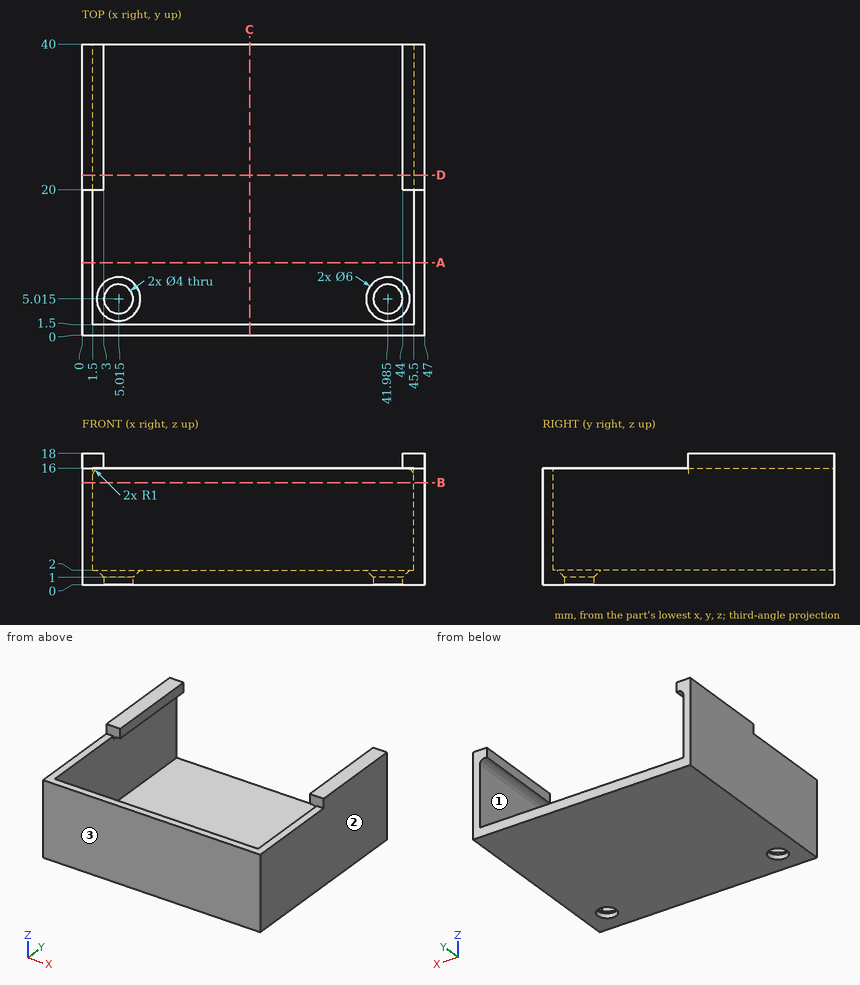
Design review of the part shown in the three views and the two pictorial views. Dimensions are in mm from the part's minimum x, y and z. Round coordinates to 2 decimals unless told otherwise and drop trailing zeros. Order: outer loops, then holes, each group sorted by start corner. A loop starts at its lowest first (then second) coordinate and runs counter-clockwise, first axis right, second up. Notation, with made-up numbers: M -14,-23.5 L 37,-23.5 A20 cw 37,13.5 Z; hole C 1.5,-10 d11. An arc over 180 degrees is marked long. Put each result on its own line as item: value.
Q1. To check wall thickness, follow line 1 (X direction, y = 8.5, z = 7.75); line 2 (Z direction, x = 4.5, y = 9); line 3 (Y direction, x = 30, z = 3.25). State the ranges of each line that lie inside material, in increasing order.
Reported:
line 1: 0 to 1.5, 45.5 to 47
line 2: 0 to 2
line 3: 0 to 1.5
Q2. Insertion check: pin 1 Ø8 at (x, y) = (22, 34) entering from +Z; pin 2 Ø4 at (x, z) = (18, 12) entering from +Y; pin 3 Ø1.5 at (x, z) = (46, 17) entering from -Y. Each pin has a flat end and moves straight along its axis. Give the tip position at first contact, or say it passes through.
Reported:
pin 1: z = 2
pin 2: y = 1.5
pin 3: y = 20
Q3. Draft analysis for pull direction X (two halves, no side actions). For the marked faces 1, 2 and 3, state which applies: released by +X, released by -X, zero draft, split by the parting line, or undercut.
Reported:
face 1: undercut
face 2: released by +X
face 3: zero draft
Q4. Consider section C-C (x = 23). State the section outline as (y, z) points.
Reported:
outline: M 0,0 L 40,0 L 40,2 L 1.5,2 L 1.5,16 L 0,16 Z
Q5. Consider section B-B (z = 14). State the section outline as (x, y) points.
Reported:
outline: M 0,0 L 47,0 L 47,40 L 45.5,40 L 45.5,1.5 L 1.5,1.5 L 1.5,40 L 0,40 Z
Q6. Consider section A-A (y = 10). State the section outline as (x, z) points, and give its area (3 significant figures).
Reported:
outline: M 0,0 L 47,0 L 47,16 L 45.5,16 L 45.5,2 L 1.5,2 L 1.5,16 L 0,16 Z
area: 136 mm²
Q7. Consider section D-D (y = 22). State the section outline as (x, z) points.
Reported:
outline: M 0,0 L 47,0 L 47,18 L 44,18 L 44,16 L 44.5,16 A1 cw 45.5,15 L 45.5,2 L 1.5,2 L 1.5,15 A1 cw 2.5,16 L 3,16 L 3,18 L 0,18 Z
